Part model, mm, in its own coordinate system. A direction names the side the tool comes from. Round coordinates to 2 decimals unless told otherwise and drop trailing zeros. Loops run counter-clockwise (first coordinate to the right, second up) from the corner with the lowest first, then second, coordinate; pieces in that order, holes last. Notation, with made-up numbers: M 24,31.25 L 73,31.25 A19 ccw 73,46.25 Z; hole C 34.25,74 d10. An arc over 180 degrees is marked long. Put each result on its own line as item: value. Start each with the question number.
1) Which spindle directions (+Z, -Z, +X, -X, +Y, -Y) get a long thin tool onto all of the face, cutting with end or side? Do faces 1 (the flat face through (-38.489, -31.823, 26.185)), 2 (the flat face through (-9, 31.062, 13)). Say none if no direction does.
2) Slice it at C-C on x = 13. Give the cut face in (y, z).
3) Slice it at B-B on y = -3. Give the cut face in (x, z), then the cut area to 3 significant figures.
4) Slice it at A-A on z = 8.5. Give the cut face in (x, y).
5) Pull direction Y, two halves, no side cores. Call faces 3 (the flat face through (-9.447, -34.952, 27.402)), 4 (the flat face through (20.743, -32.173, 12.666)), 5 (the flat face through (21.917, 28.597, 13.023)): +Y half, -Y half, draft (parallel to the pull), parting line (faces both ways), or undercut.
6) Probe line 1 along X through (y, z) = (11, 18.5); line 2 along Y through (x, z) = (13, 19.25); line 3 along Z through (x, y) = (-0.5, -23). List the from-to ranges inside material, lowest first.
```python
from build123d import *

# Parameters (mm, degrees)
F0_W     = 67
F0_H     = 67
F1_DEPTH = 28.416
F2_SIZE  = 5
F3_SIZE  = 2
F4_T     = -1.75


with BuildPart() as f1:
    # F0 (on Top) → F1 (new body)
    with BuildSketch(Plane.XY):
        with Locations((-9.047817, -2.437839)):
            Rectangle(F0_W, F0_H)
    extrude(amount=F1_DEPTH)

    # F2
    f2_edges = [f1.edges().sort_by_distance(p)[0] for p in [
        (-42.547817, -35.937839, 14.208),
        (24.452183, -35.937839, 14.208),
        (24.452183, 31.062161, 14.208),
        (-42.547817, 31.062161, 14.208),
    ]]
    chamfer(f2_edges, length=F2_SIZE)

    # F3
    f3_edges = [f1.edges().sort_by_distance(p)[0] for p in [
        (-9.047817, 31.062161, 28.416),
        (21.952183, 28.562161, 28.416),
        (-40.047817, 28.562161, 28.416),
        (24.452183, -2.437839, 28.416),
        (-42.547817, -2.437839, 28.416),
        (21.952183, -33.437839, 28.416),
        (-40.047817, -33.437839, 28.416),
        (-9.047817, -35.937839, 28.416),
    ]]
    chamfer(f3_edges, length=F3_SIZE)

    # F4
    f4_openings = [f1.faces().sort_by_distance(p)[0] for p in [
        (-9.047817, -2.437839, 0),
    ]]
    offset(amount=F4_T, openings=f4_openings)


solid = f1.part
```
Recorded:
1. face 1: -Z
1. face 2: +Z, -Z, +X, -X, +Y
2. outline: M -35.94,0 L -34.19,0 L -34.19,25.69 L -33.21,26.67 L 28.34,26.67 L 29.31,25.69 L 29.31,0 L 31.06,0 L 31.06,26.42 L 29.06,28.42 L -33.94,28.42 L -35.94,26.42 Z
3. outline: M -42.55,0 L -40.8,0 L -40.8,25.69 L -39.82,26.67 L 21.73,26.67 L 22.7,25.69 L 22.7,0 L 24.45,0 L 24.45,26.42 L 22.45,28.42 L -40.55,28.42 L -42.55,26.42 Z
3. area: 208 mm2
4. outline: M -42.55,-30.94 L -37.55,-35.94 L 19.45,-35.94 L 24.45,-30.94 L 24.45,26.06 L 19.45,31.06 L -37.55,31.06 L -42.55,26.06 Z; hole M -40.8,-30.21 L -36.82,-34.19 L 18.73,-34.19 L 22.7,-30.21 L 22.7,25.34 L 18.73,29.31 L -36.82,29.31 L -40.8,25.34 Z
5. face 3: -Y half
5. face 4: undercut
5. face 5: +Y half
6. line 1: x = -42.55 to -40.8, 22.7 to 24.45
6. line 2: y = -35.94 to -34.19, 29.31 to 31.06
6. line 3: z = 26.67 to 28.42
